```python
from build123d import *

# Parameters (mm, degrees)
F1_DEPTH = 12
F3_D     = 3
F3_DEPTH = 25
F4_R     = 3
F5_R     = 2


with BuildPart() as f1:
    # F0 (on Top) → F1 (new body)
    with BuildSketch(Plane.XY):
        Polygon((17.880361, 2.160541), (5.880361, 2.160541), (5.880361, -1.839459), (21.880361, -1.839459), (21.880361, 8.660541), (63.880361, 8.660541), (63.880361, -1.839459), (79.880361, -1.839459), (79.880361, 2.160541), (67.880361, 2.160541), (67.880361, 12.660541), (17.880361, 12.660541), align=None)
    extrude(amount=F1_DEPTH)

    # F3
    with Locations(Plane.XZ.offset(1.839459)):
        with Locations((11.880361, 6), (73.880361, 6)):
            Hole(F3_D / 2, depth=F3_DEPTH)

    # F4
    f4_edges = [f1.edges().sort_by_distance(p)[0] for p in [
        (67.880361, 2.160541, 6),
        (79.880361, 0.160541, 12),
        (79.880361, 0.160541, 0),
        (5.880361, 0.160541, 0),
        (17.880361, 2.160541, 6),
        (5.880361, 0.160541, 12),
    ]]
    fillet(f4_edges, radius=F4_R)

    # F5
    f5_edges = [f1.edges().sort_by_distance(p)[0] for p in [
        (17.880361, 12.660541, 6),
        (67.880361, 12.660541, 6),
    ]]
    fillet(f5_edges, radius=F5_R)


solid = f1.part
```
Verification items for the finished model (mm, model axes). A direction names the side the tool comes from. Coordinates: 2 decimals unless noted, no trailing zeros. Loops run counter-clockwise (first coordinate to the right, second up) from the corner with the lowest first, then second, coordinate; pieces in that order, holes last. Notation, with made-up numbers: (-28.75, 7) -> (8.25, 7) arc R23 cw to (8.25, 26) -> close; hole circle Ø11 at (37, 61.5). An arc over 180 degrees is marked (long way). Put each result on its own line as item: value.
1. Section check A-A, the plane y = 0. Record the boundary of the cut face in (x, z), then the cut area to 3 significant figures.
Result set:
outline: (5.88, 3) arc R3 ccw to (8.88, 0) -> (21.88, 0) -> (21.88, 12) -> (8.88, 12) arc R3 ccw to (5.88, 9) -> close; (63.88, 0) -> (76.88, 0) arc R3 ccw to (79.88, 3) -> (79.88, 9) arc R3 ccw to (76.88, 12) -> (63.88, 12) -> close; hole circle Ø3 at (11.88, 6); hole circle Ø3 at (73.88, 6)
area: 362 mm^2
2. Mould release check, pull along X, two halves, no side actions. Record for faces 1 (the face through (63.88, 3, 6)), 2 (the face through (42, 9, 0)), 3 (the face through (6.78, 0.13, 0.86)), 4 (the face through (13.38, 0.19, 6.07)): pulls with the +X half, pulls with the -X half, needs draft (parallel to the pull), parting line crosses it, or undercut.
Result set:
face 1: undercut
face 2: needs draft
face 3: pulls with the -X half
face 4: undercut
3. Gauge pin test, flat ends, axial feed: P1, Ø1, axis at x = 63, y = 2, coming from the -Z side; P2, Ø4.5, axis at x = 10, z = 9, coming from the +Y side; P3, Ø3, axis at y = 9, z = 7.5, coming from the +X side; P4, Ø1.6, axis at y = 7, z = 8, coming from the -X side. Record the tip position at first contact, or that the pin passes through.
Result set:
P1: passes through
P2: stops at y = 2.16
P3: stops at x = 67.88
P4: stops at x = 17.88
4. Section check C-C, the plane y = 7.5. Record the boundary of the cut face in (x, z).
Result set:
outline: (17.88, 0) -> (21.88, 0) -> (21.88, 12) -> (17.88, 12) -> close; (63.88, 0) -> (67.88, 0) -> (67.88, 12) -> (63.88, 12) -> close
5. Section check B-B, the plane z = 6. Record the boundary of the cut face in (x, y), then the cut area to 3 significant figures.
Result set:
outline: (5.88, -1.84) -> (10.38, -1.84) -> (10.38, 2.16) -> (5.88, 2.16) -> close; (13.38, -1.84) -> (21.88, -1.84) -> (21.88, 8.66) -> (63.88, 8.66) -> (63.88, -1.84) -> (72.38, -1.84) -> (72.38, 2.16) -> (70.88, 2.16) arc R3 cw to (67.88, 5.16) -> (67.88, 10.66) arc R2 ccw to (65.88, 12.66) -> (19.88, 12.66) arc R2 ccw to (17.88, 10.66) -> (17.88, 5.16) arc R3 cw to (14.88, 2.16) -> (13.38, 2.16) -> close; (75.38, -1.84) -> (79.88, -1.84) -> (79.88, 2.16) -> (75.38, 2.16) -> close
area: 358 mm^2
6. Tool access check on faces 5 (the face through (17.88, 8, 6)), 6 (the face through (43, 8.661, 6)), 7 (the face through (5.88, 0, 6)), 8 (the face through (76, 2.161, 6)). Record the directions out of +Z, -Z, +X, -X, +Y, -Y that give a thin tool (end or side, any length) a straight path to the whole face; none if there is none.
Result set:
face 5: +Z, -Z, -X, +Y
face 6: +Z, -Z, -Y
face 7: +Z, -Z, -X, +Y, -Y
face 8: +Z, -Z, +X, +Y
7. Section check D-D, the plane x = 23.5. Record the boundary of the cut face in (y, z), then the cut area to 3 significant figures.
Result set:
outline: (8.66, 0) -> (12.66, 0) -> (12.66, 12) -> (8.66, 12) -> close
area: 48.0 mm^2
8. Thickness scan on line 1 (X direction, y = 6.5, z = 5.25); line 2 (Y direction, x = 50, z = 2.75); line 3 (Y direction, x = 10, z = 8.5). Record the ranges inside material, lowest first.
Result set:
line 1: x = 17.88 to 21.88, 63.88 to 67.88
line 2: y = 8.66 to 12.66
line 3: y = -1.84 to 2.16
